Verification items for the finished model (mm, model axes). Face numbers are marked on the shaded views. A direction names the side the tool comes from. Round coordinates to 2 decimals unless told otherwise and drop trailing zeros. Order: outer loops, then holes, each group sorted by start corner. A loop starts at its lowest first (then second) coordinate and runs counter-clockwise, first axis right, second up. Notation, with made-up numbers: M -40,1.25 L 1,1.25 A26 cw 1,21.25 Z; hole C 34,-19 d6. An arc over 180 degrees is marked long. Use one line per item in the form item = value. Start each with the question number.
Item 1: Cross-section at A-A on x = -14. Enter the section's corners in (y, z), then the cut area to 3 significant figures.
Item 2: Tool access check on the marked faces 1 and 2. Record the directions out of +Z, -Z, +X, -X, +Y, -Y that give a thin tool (end or side, any length) a straight path to the whole face; none if there is none.
Item 3: Thickness scan on probe 1 along Y at (x, z) = (-15, 1); probe 2 along Z at (x, y) = (-21, -2.3); probe 3 along Z at (x, y) = (21, -2.15). Record the ranges inside material, lowest first. Write a range as [from, to].
Item 4: Cross-section at C-C on z = -1. Enter the section's corners in (x, y), then the cut area to 3 significant figures.
Item 5: Go/stop test with flat-tipped pins: pin 1 Ø12 at (x, z) = (-8.5, 8.5) entering from -Y; pin 2 Ø4 at (x, z) = (10, 17.5) entering from -Y; pin 3 Ø6 at (x, z) = (0, 2) entering from -Y. Record where each tip stops, or that it passes through.
Item 6: Cross-section at B-B on x = 17.5. Enter the section's corners in (y, z), then the cut area to 3 significant figures.
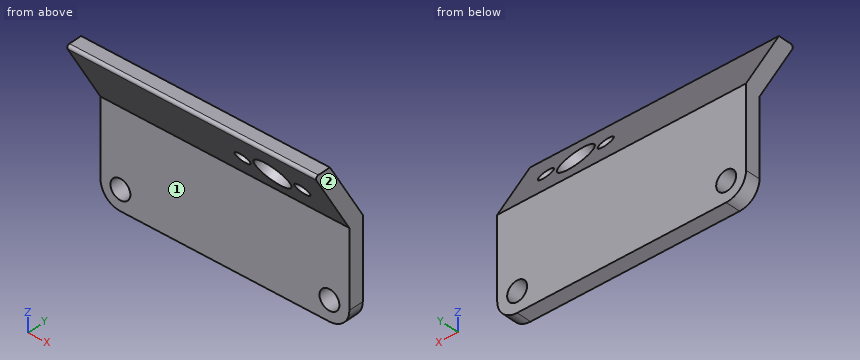
from build123d import *

# Parameters (mm, degrees)
F0_W     = 50
F0_H     = 20
F0_R     = 2
F1_DEPTH = 3
F2_R     = 4
F4_DEPTH = 50
F6_DEPTH = 25
F7_R     = 0.5


with BuildPart() as f1:
    # F0 (on Front) → F1 (new body)
    with BuildSketch(Plane.XZ):
        Rectangle(F0_W, F0_H)
        with Locations((-21, -6)):
            Circle(F0_R, mode=Mode.SUBTRACT)
        with Locations((21, -6)):
            Circle(F0_R, mode=Mode.SUBTRACT)
    extrude(amount=F1_DEPTH)

    # F2
    f2_edges = [f1.edges().sort_by_distance(p)[0] for p in [
        (-25, -1.5, -10),
        (25, -1.5, -10),
    ]]
    fillet(f2_edges, radius=F2_R)

    # F3 (on face) → F4 (join)
    with BuildSketch(Plane.YZ.offset(25)):
        Polygon((0, 10), (-7.3274360099, 22.6914914583), (-10.791537625, 22.6914914583), (-3, 9.1961524227), (-3, 10), align=None)
    extrude(amount=-F4_DEPTH)

    # F5 (on face) → F6 (cut)
    with BuildSketch(Plane(origin=(0, 4.3301270189, 2.5), x_dir=(-1, 0, 0), z_dir=(0, 0.8660254038, 0.5))):
        with BuildLine():
            Line((-16, 15.9876900477), (-9, 15.9876900477))
            ThreePointArc((-9, 15.9876900477), (-12.5, 19.4876900477), (-16, 15.9876900477))
        make_face()
        with BuildLine():
            ThreePointArc((-20, 15.9876900477), (-18.5, 14.4876900477), (-17, 15.9876900477))
            Line((-17, 15.9876900477), (-20, 15.9876900477))
        make_face()
        with BuildLine():
            Line((-20, 15.9876900477), (-17, 15.9876900477))
            ThreePointArc((-17, 15.9876900477), (-18.5, 17.4876900477), (-20, 15.9876900477))
        make_face()
        with BuildLine():
            ThreePointArc((-5, 15.9876900477), (-6.5, 17.4876900477), (-8, 15.9876900477))
            Line((-8, 15.9876900477), (-5, 15.9876900477))
        make_face()
        with BuildLine():
            Line((-5, 15.9876900477), (-8, 15.9876900477))
            ThreePointArc((-8, 15.9876900477), (-6.5, 14.4876900477), (-5, 15.9876900477))
        make_face()
        with BuildLine():
            ThreePointArc((-16, 15.9876900477), (-12.5, 12.4876900477), (-9, 15.9876900477))
            Line((-9, 15.9876900477), (-16, 15.9876900477))
        make_face()
    extrude(amount=-F6_DEPTH, mode=Mode.SUBTRACT)

    # F7
    f7_edges = [f1.edges().sort_by_distance(p)[0] for p in [
        (0, -10.791538, 22.691491),
    ]]
    fillet(f7_edges, radius=F7_R)


solid = f1.part
Output values:
q1.outline = M -10.36,21.94 L -3,9.2 L -3,-10 L 0,-10 L 0,10 L -7.33,22.69 L -9.93,22.69 A0.5 ccw Z
q1.area = 104 mm2
q2.face_1 = -Z, +X, -X, -Y
q2.face_2 = +Z, -Z, +X, +Y, -Y
q3.probe_1 = [-3, 0]
q3.probe_2 = [-10, -8], [-4, 13.98]
q3.probe_3 = [-10, -8], [-4, 13.72]
q4.outline = M -25,-3 L 25,-3 L 25,0 L -25,0 Z
q4.area = 150 mm2
q5.pin_1 = -6.06
q5.pin_2 = -8.95
q5.pin_3 = -3
q6.outline = M -10.36,21.94 L -6.82,15.81 L -4.22,17.31 L -7.33,22.69 L -9.93,22.69 A0.5 ccw Z; M -5.7,13.88 L -3,9.2 L -3,-10 L 0,-10 L 0,10 L -3.1,15.38 Z
q6.area = 97.3 mm2
